For this review, use the dimensioned drawing (mm, ordinates from the lowest corner) and the shaded views. A direction names the side the tool comes from. Coordinates: 2 decimals unless noted, no trailing zeros. Loops run counter-clockwise (first coordinate to the right, second up) from the corner with the lowest first, then second, coordinate; pieces in that order, holes last. Notation, with made-up numbers: M 6.25,-40 L 49.25,-40 A15 ccw 49.25,-25 Z; hole C 83.25,54 d10. An arc over 180 degrees is marked long. Write item = value, one per line.
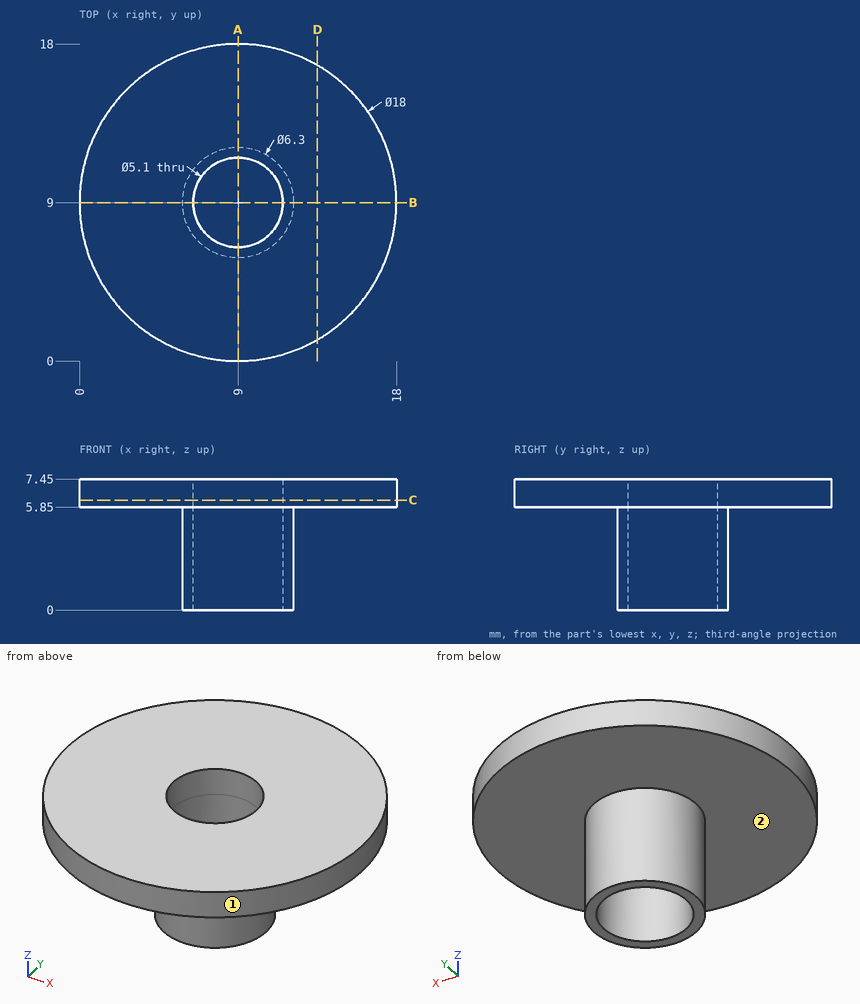
Q1. Add section C-C (z = 6.25). Write out the cut boundary in (x, y), and give its area (3 significant figures).
Solved:
outline = C 9,9 d18; hole C 9,9 d5.1
area = 234 mm²
Q2. For pin 1 Ø2 at (x, z) = (15, 3.5) entering from +Y; pin 2 Ø1.5 at (x, z) = (10.5, 5) entering from +Y; pin 3 Ø2 at (x, y) = (11.5, 13.5) entering from -Z; pin 4 Ø1 at (y, z) = (14, 6) entering from -X, all flat-tipped, find the tip position at first contact; note any pin that passes through.
Solved:
pin_1 = through
pin_2 = 12.06
pin_3 = 5.85
pin_4 = 1.21
Q3. For line 1 along Y through (x, z) = (9, 6.7); line 2 along Z through (x, y) = (17.5, 9.5); line 3 along X through (y, z) = (9, 4), list the stretches that pass through material, from the lowest coordinate up.
Solved:
line_1 = 0 to 6.45, 11.55 to 18
line_2 = 5.85 to 7.45
line_3 = 5.85 to 6.45, 11.55 to 12.15
Q4. Machinability: for the marked faces 1 and 2, which of the approach directions +Z, -Z, +X, -X, +Y, -Y give a long, thin tool a straight path to every point of the face, cutting with its end or side? Answer none if there is none.
Solved:
face_1 = +Z, -Z
face_2 = -Z
Q5. Add section A-A (x = 9). Write out the cut boundary in (y, z), and give its area (3 significant figures).
Solved:
outline = M 0,5.85 L 5.85,5.85 L 5.85,0 L 6.45,0 L 6.45,7.45 L 0,7.45 Z; M 11.55,0 L 12.15,0 L 12.15,5.85 L 18,5.85 L 18,7.45 L 11.55,7.45 Z
area = 27.7 mm²
Q6. Add section D-D (x = 13.5). Write out the cut boundary in (y, z), and give its area (3 significant figures).
Solved:
outline = M 1.21,5.85 L 16.79,5.85 L 16.79,7.45 L 1.21,7.45 Z
area = 24.9 mm²
